The model under review builds one solid part; all positions refer to its coordinate system, in mm. Face numbers are marked on the shaded views. A direction names the side the tool comes from. Give positions to 0.01 mm unless a question says otherwise; leave off trailing zeros. Write each loop counter-clockwise with the first axis right and the second up, starting at its lowest first coordinate (ties: lowest second). Pieces come first, ordered by that corner, then holes. Notation, with made-up numbers: (42.5, 30.5) - (93.5, 30.5) arc R32 ccw to (93.5, 56.5) - close; hole circle Ø4 at (-15.75, 56.25). An arc over 180 degrees is marked (long way). Write item = value, one per line.
```python
from build123d import *

# Parameters (mm, degrees)
SKETCH1_W                = 50
SKETCH1_H                = 50
BOSS_EXTRUDE1_DEPTH      = 25
CUT_EXTRUDE2_DEPTH       = 76
CUT_EXTRUDE3_DEPTH       = 22
CHAMFER1_SIZE            = 4
CHAMFER2_SIZE            = 1.5
BOSS_EXTRUDE2_DEPTH      = 7
BOSS_EXTRUDE2_DEPTH_BACK = 10
SKETCH6_W                = 1
SKETCH6_H                = 7
SKETCH7_W                = 1.8
SKETCH7_H                = 1.8
CUT_EXTRUDE4_DEPTH       = 78.614431648


with BuildPart() as part:
    # Sketch1 → Boss-Extrude1 (new body)
    with BuildSketch(Plane.XY):
        with Locations((25, 25)):
            Rectangle(SKETCH1_W, SKETCH1_H)
    extrude(amount=BOSS_EXTRUDE1_DEPTH)

    # Sketch3 → Cut-Extrude2 (cut, through all)
    with BuildSketch(Plane.XZ):
        Polygon((36, 29.556349186), (29.556349186, 36), (20.443650814, 36), (14, 29.556349186), (14, 20.443650814), (20.443650814, 14), (29.556349186, 14), (36, 20.443650814), align=None)
    extrude(amount=-CUT_EXTRUDE2_DEPTH, mode=Mode.SUBTRACT)

    # Sketch5 → Cut-Extrude3 (cut)
    with BuildSketch(Plane.XY.offset(25)):
        Polygon((4, 33.69848481), (4, 16.30151519), (16.30151519, 4), (33.69848481, 4), (46, 16.30151519), (46, 33.69848481), (33.69848481, 46), (16.30151519, 46), align=None)
    extrude(amount=-CUT_EXTRUDE3_DEPTH, mode=Mode.SUBTRACT)

    # Chamfer1
    chamfer1_edges = [part.edges().sort_by_distance(p)[0] for p in [
        (39.849242405, 39.849242405, 3),
        (39.849242405, 10.150757595, 3),
        (10.150757595, 39.849242405, 3),
        (25, 46, 3),
        (25, 4, 3),
        (10.150757595, 10.150757595, 3),
        (46, 25, 3),
        (4, 25, 3),
    ]]
    chamfer(chamfer1_edges, length=CHAMFER1_SIZE)

    # Chamfer2
    chamfer2_edges = [part.edges().sort_by_distance(p)[0] for p in [
        (50, 25, 25),
        (43, 50, 25),
        (43, 0, 25),
        (7, 50, 25),
        (14, 3.150757595, 25),
        (36, 46.849242405, 25),
        (36, 50, 22.721825407),
        (14, 50, 22.721825407),
        (36, 0, 22.721825407),
        (14, 0, 22.721825407),
        (17.221825407, 0, 17.221825407),
        (32.778174593, 0, 17.221825407),
        (32.778174593, 50, 17.221825407),
        (17.221825407, 50, 17.221825407),
        (0, 25, 25),
        (25, 50, 0),
        (50, 25, 0),
        (14, 46.849242405, 25),
        (36, 3.150757595, 25),
        (25, 0, 0),
        (41, 38.69848481, 25),
        (41, 11.30151519, 25),
        (46, 25, 25),
        (9, 11.30151519, 25),
        (9, 38.69848481, 25),
        (4, 25, 25),
        (0, 25, 0),
        (7, 0, 25),
        (50, 50, 12.5),
        (50, 0, 12.5),
        (0, 0, 12.5),
    ]]
    chamfer(chamfer2_edges, length=CHAMFER2_SIZE)

    # Sketch6 → Boss-Extrude2 (add, two sides: drawn at the far end of the back side and taken through both)
    with BuildSketch(Plane.XY.offset(25).offset(-BOSS_EXTRUDE2_DEPTH_BACK)):
        with Locations((49.5, 25)):
            Rectangle(SKETCH6_W, SKETCH6_H)
    extrude(amount=BOSS_EXTRUDE2_DEPTH + BOSS_EXTRUDE2_DEPTH_BACK)

    # Sketch7 → Cut-Extrude4 (cut, through all)
    with BuildSketch(Plane(origin=(50, 0, 0), x_dir=(0, 0, -1), z_dir=(1, 0, 0))):
        with Locations((-28.6, 25)):
            Rectangle(SKETCH7_W, SKETCH7_H)
    extrude(amount=-CUT_EXTRUDE4_DEPTH, mode=Mode.SUBTRACT)


solid = part.part
```
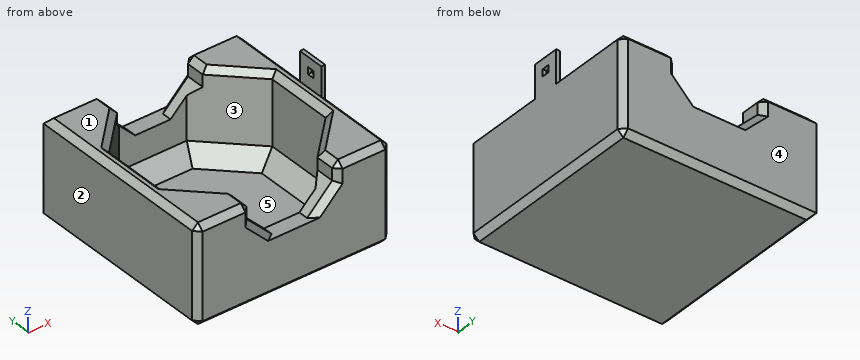
1. For line 1 (X direction, y = 27.5, z = 9); line 2 (Z direction, x = 42, y = 45); line 3 (Z direction, x = 32.5, y = 39.5), list the stretches that pass through material, from the lowest coordinate up. Write a range as from..to.
Findings below:
line_1 = 0..4, 46..50
line_2 = 0..25
line_3 = 0..3
2. Insertion check: P1, Ø0.8, axis at x = 49.5, y = 25.5, coming from the -Z side; P2, Ø10, axis at x = 11, y = 44, coming from the +Z side; P3, Ø3.5, axis at x = 9.5, y = 36, coming from the +Z side. Each pin has a flat end and moves straight along its axis. Give the tip position at first contact, or say it passes through.
Findings below:
P1 = 0.6
P2 = 25
P3 = 6.49
3. Take a section at B-B on z = 17.5. Give the boundary of the cut face in (x, y), and give its area (3 significant figures).
Findings below:
outline = (0, 1.5) - (1.5, 0) - (14.82, 0) - (16.94, 1.5) - (16.94, 4) - (16.3, 4) - (4, 16.3) - (4, 33.7) - (16.3, 46) - (16.94, 46) - (16.94, 48.5) - (14.82, 50) - (0, 50) - close; (33.06, 1.5) - (35.18, 0) - (48.5, 0) - (50, 1.5) - (50, 48.5) - (48.5, 50) - (35.18, 50) - (33.06, 48.5) - (33.06, 46) - (33.7, 46) - (46, 33.7) - (46, 16.3) - (33.7, 4) - (33.06, 4) - close
area = 900 mm²
4. Take a section at A-A on z = 9. Give the boundary of the cut face in (x, y), and give its area (3 significant figures).
Findings below:
outline = (0, 1.5) - (1.5, 0) - (48.5, 0) - (50, 1.5) - (50, 48.5) - (48.5, 50) - (0, 50) - close; hole (4, 16.3) - (16.3, 4) - (33.7, 4) - (46, 16.3) - (46, 33.7) - (33.7, 46) - (16.3, 46) - (4, 33.7) - close
area = 1,040 mm²
5. Take a section at C-C on y = 37. Give the boundary of the cut face in (x, z), and give its area (3 significant figures).
Findings below:
outline = (0, 1.5) - (1.5, 0) - (48.5, 0) - (50, 1.5) - (50, 23.5) - (48.5, 25) - (44.82, 25) - (42.7, 23.5) - (42.7, 7) - (37.04, 3) - (12.96, 3) - (7.3, 7) - (7.3, 23.5) - (5.18, 25) - (1.5, 25) - (0, 23.5) - close
area = 486 mm²
6. Take a section at D-D on x = 40. Give the boundary of the cut face in (y, z), and give its area (3 significant figures).
Findings below:
outline = (0, 1.5) - (1.5, 0) - (48.5, 0) - (50, 1.5) - (50, 23.5) - (48.5, 25) - (41.82, 25) - (39.7, 23.5) - (39.7, 7) - (34.04, 3) - (15.96, 3) - (10.3, 7) - (10.3, 23.5) - (8.18, 25) - (1.5, 25) - (0, 23.5) - close
area = 618 mm²
7. Draft analysis for pull direction X (two halves, no side actions). For the marked faces 1, 2 and 3, state which applies: +X half, -X half, draft (parallel to the pull), parting line (faces both ways), or undercut.
Findings below:
face_1 = draft
face_2 = -X half
face_3 = undercut
8. Machinability: for the marked faces 4 and 5, which of the approach directions +Z, -Z, +X, -X, +Y, -Y give a long, thin tool a straight path to every point of the face, cutting with its end or side? Answer none if there is none.
Findings below:
face_4 = +Z, -Z, +X, -X, +Y
face_5 = +Z
